Study the drawing (mm; zero at the part's minimum x, y, z) and answer. A direction names the side the tool comes from. Round coordinates to 2 decimals unless told otherwise and drop trailing zeros. Order: outer loops, then holes, each group sorted by start corner. A loop starts at its lowest first (then second) coordinate and runs counter-clockwise, first axis right, second up. Notation, with made-up numbers: (73.5, 9.5) -> (87.5, 9.5) arc R10 ccw to (87.5, 21.5) -> close; hole circle Ø9 at (20.5, 11.25). An arc over 180 degrees is marked (long way). Use one line per item in the form item = value.
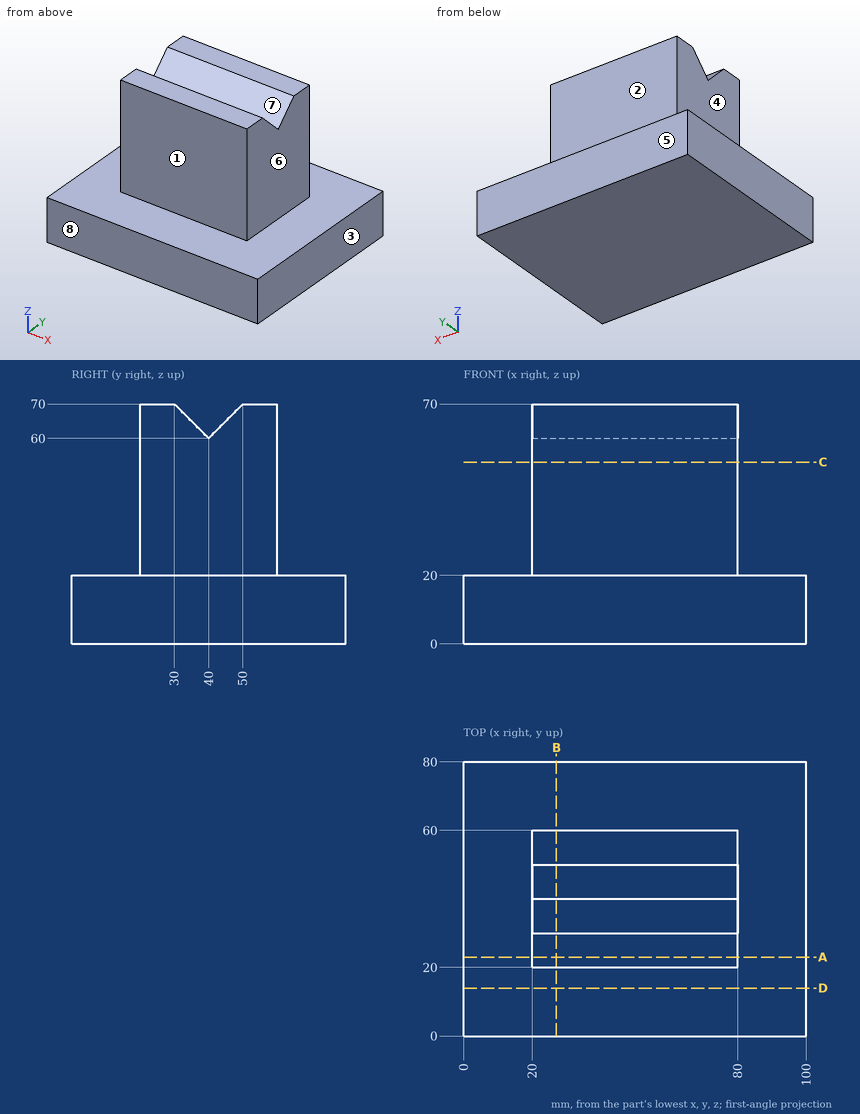
Item 1: For the marked faces 1, 2, 3 and 4, determine the directions among +Z, -Z, +X, -X, +Y, -Y from which every point of the face is accessible in a straight line to the end or side of a thin tool.
Findings:
face_1 = +Z, +X, -X, -Y
face_2 = +Z, +X, -X, +Y
face_3 = +Z, -Z, +X, +Y, -Y
face_4 = +Z, -X, +Y, -Y
Item 2: Flat-ended cylindrical pins translate along their axes: P1, Ø3, axis at x = 47, z = 57.5, coming from the -Y side; P2, Ø6, axis at x = 69, z = 23.5, coming from the +Y side; P3, Ø12, axis at x = 36, y = 68.5, coming from the +Z side; P4, Ø2, axis at x = 29.5, y = 33, coming from the -Z side. Find the tip coordinate at first contact, or state that the pin passes through.
Findings:
P1 = 20
P2 = 60
P3 = 20
P4 = 0
Item 3: The part is cut by section C-C, the plane z = 53. Give the vertices of the cut face in (x, y), and give its area (3 significant figures).
Findings:
outline = (20, 20) -> (80, 20) -> (80, 60) -> (20, 60) -> close
area = 2,400 mm^2
Item 4: The part is cut by section A-A, the plane y = 23. Give the vertices of the cut face in (x, z), and give its area (3 significant figures).
Findings:
outline = (0, 0) -> (100, 0) -> (100, 20) -> (80, 20) -> (80, 70) -> (20, 70) -> (20, 20) -> (0, 20) -> close
area = 5,000 mm^2
Item 5: The part is cut by section B-B, the plane x = 27. Give the vertices of the cut face in (y, z), and give its area (3 significant figures).
Findings:
outline = (0, 0) -> (80, 0) -> (80, 20) -> (60, 20) -> (60, 70) -> (50, 70) -> (40, 60) -> (30, 70) -> (20, 70) -> (20, 20) -> (0, 20) -> close
area = 3,500 mm^2
Item 6: The part is cut by section D-D, the plane y = 14. Give the vertices of the cut face in (x, z).
Findings:
outline = (0, 0) -> (100, 0) -> (100, 20) -> (0, 20) -> close
Item 7: Determine the mould class of the marked faces 5, 6, 7 and 8 for opening direction Y: released by +Y, released by -Y, zero draft, split by the parting line, or undercut.
Findings:
face_5 = released by +Y
face_6 = zero draft
face_7 = undercut
face_8 = released by -Y
Item 8: Consider line 1 along Y through (x, z) = (21, 58); line 2 along Z through (x, y) = (93, 66); line 3 along X through (y, z) = (55, 50.5). Determine where each line is inside the solid, lowest interval first.
Findings:
line_1 = 20 to 60
line_2 = 0 to 20
line_3 = 20 to 80
